Input: dimensioned drawing with shaded views. Units: mm. Origin: part minimum x, y, z. A direction names the side the tool comes from. Coordinates: 2 decimals unless noted, no trailing zeros. Write each loop counter-clockwise with the first axis right and the second up, starting at its lowest first coordinate (ties: lowest second). Pieces come first, ordered by that corner, then holes. Notation, with made-up numbers: (30.5, -13.5) - (85.5, -13.5) arc R19 ccw to (85.5, 17.5) - close; hole circle Ø6 at (35, 87). An arc over 180 degrees is marked (long way). One line per question, with ' | ' between items.
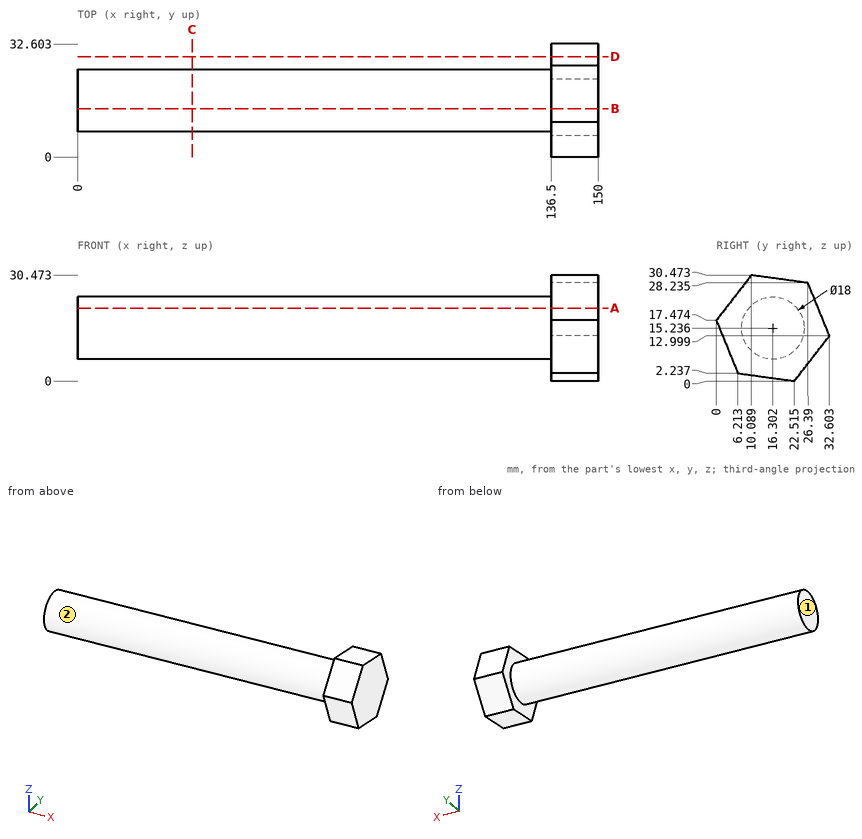
Item 1: Ray query, line 1 along X through (y, z) = (12, 3.5); line 2 along Z through (x, y) = (63, 15); line 3 along Y through (x, z) = (28, 11.5) (1 decimal). Return the intervals inside material, ascending. Write a range as [from, to].
Check sheet entries:
line 1: [136.5, 150] | line 2: [6.33, 24.14] | line 3: [8.1, 24.5]
Item 2: Cut plane D-D on y = 29. Return loops of the section in (x, z) (1 decimal), and give its area (3 significant figures).
Check sheet entries:
outline: (136.5, 8.4) - (150, 8.4) - (150, 21.8) - (136.5, 21.8) - close | area: 182 mm²
Item 3: Pin query (flat end, axial travel): pin 1 Ø1.5 at (x, z) = (21, 14) entering from -Y (1 decimal); pin 2 Ø6 at (x, y) = (50, 6.5) entering from +Z; pin 3 Ø3 at (x, y) = (78.5, 21.5) entering from +Z. Return the tip coordinate at first contact, or that it passes through.
Check sheet entries:
pin 1: y = 7.3 | pin 2: z = 21.13 | pin 3: z = 23.44
Item 4: Access query for the marked faces 1 and 2. Directions: +Z, -Z, +X, -X, +Y, -Y. A direction counts if a zero-diameter tool reaches every point of the face in a straight line with its end or side. Return the directions, or none.
Check sheet entries:
face 1: +Z, -Z, -X, +Y, -Y | face 2: -X
Item 5: Cut plane B-B on y = 14. Return loops of the section in (x, z) (1 decimal), and give its area (3 significant figures).
Check sheet entries:
outline: (0, 6.5) - (136.5, 6.5) - (136.5, 1.2) - (150, 1.2) - (150, 29.9) - (136.5, 29.9) - (136.5, 23.9) - (0, 23.9) - close | area: 2,760 mm²
Item 6: Cut plane C-C on x = 33. Return loops of the section in (y, z).
Check sheet entries:
outline: circle Ø18 at (16.3, 15.24)
Item 7: Cut plane A-A on z = 21. Return loops of the section in (x, y).
Check sheet entries:
outline: (0, 9.39) - (136.5, 9.39) - (136.5, 2.74) - (150, 2.74) - (150, 29.34) - (136.5, 29.34) - (136.5, 23.21) - (0, 23.21) - close
